For this review, take the finished solid that the model builds, in its own axes (mm). A direction names the side the tool comes from. Coordinates: 2 decimals unless noted, no trailing zeros. Loops run counter-clockwise (first coordinate to the right, second up) from the corner with the lowest first, then second, coordinate; pieces in that order, holes last. Notation, with made-up numbers: (10.25, 49.25) - (31.25, 49.25) arc R7 ccw to (31.25, 61.25) - close; hole circle Ø2 at (45.5, -26). An arc over 180 degrees is marked (long way). Use one line per item in the form item = value. Start each with the question number.
1. Add section B-B on z = 0.3. Give the boundary of the cut face in (x, y).
2. Add section C-C on x = 1.5. Give the boundary of the cut face in (y, z), and give its area (3 significant figures).
3. Add section D-D on y = 1.3. Give the boundary of the cut face in (x, z).
4. To check wall thickness, follow probe 1 along X at (y, z) = (0.9, 3.3); probe 2 along X at (y, z) = (1.05, 3.7); probe 3 along Y at (x, z) = (-0.5, 0.65). State the ranges of each line that lie inside material, in increasing order.
5. For pin 1 Ø1 at (x, z) = (-0.5, 2.5) entering from +Y, flat-tipped, find the tip position at first contact; note if it passes through.
6. Add section A-A on y = 1.9. Give the boundary of the cut face in (x, z).
7. Machinability: for faces 1 (the face through (-1.13, 0.67, 2.46)), 2 (the face through (0, 1, 5)), which of the approach directions +Z, -Z, +X, -X, +Y, -Y give a long, thin tool a straight path to every point of the face, cutting with its end or side? Answer none if there is none.
```python
from build123d import *

# Parameters (mm, degrees)
ESBO_O1_R                  = 0.8
RESSALTO_EXTRUS_O1_DEPTH   = 5
RESSALTO_EXTRUS_O1_2_DEPTH = 5
RESSALTO_EXTRUS_O1_3_DEPTH = 5
RESSALTO_EXTRUS_O1_4_DEPTH = 5
ESBO_O2_R                  = 0.8
ESBO_O2_W                  = 5
ESBO_O2_H                  = 0.5
RESSALTO_EXTRUS_O2_DEPTH   = 1


with BuildPart() as part:
    # Esbo_o1 → Ressalto-extrus_o1 (new body)
    with BuildSketch(Plane.XY):
        with Locations((-3.502077011, 1.3792577)):
            Circle(ESBO_O1_R)
    extrude(amount=RESSALTO_EXTRUS_O1_DEPTH)



with BuildPart() as body_2:
    # Esbo_o1 → Ressalto-extrus_o1 2 (new body)
    with BuildSketch(Plane.XY):
        with Locations((-1.502077011, 1.3792577)):
            Circle(ESBO_O1_R)
    extrude(amount=RESSALTO_EXTRUS_O1_2_DEPTH)


with BuildPart() as body_3:
    # Esbo_o1 → Ressalto-extrus_o1 3 (new body)
    with BuildSketch(Plane.XY):
        with Locations((0.497922989, 1.3792577)):
            Circle(ESBO_O1_R)
    extrude(amount=RESSALTO_EXTRUS_O1_3_DEPTH)


with BuildPart() as body_4:
    # Esbo_o1 → Ressalto-extrus_o1 4 (new body)
    with BuildSketch(Plane.XY):
        with Locations((2.497922989, 1.3792577)):
            Circle(ESBO_O1_R)
    extrude(amount=RESSALTO_EXTRUS_O1_4_DEPTH)


with BuildPart() as part_1:
    add(part.part)

    add(body_2.part)  # Ressalto-extrus_o2 merges body 2

    add(body_3.part)  # Ressalto-extrus_o2 merges body 3

    add(body_4.part)  # Ressalto-extrus_o2 merges body 4
    # Esbo_o2 → Ressalto-extrus_o2 (add)
    with BuildSketch(Plane(origin=(0, 0, 0), x_dir=(-1, 0, 0), z_dir=(0, 0, -1))):
        with Locations((-2.497922989, 1.3792577)):
            Circle(ESBO_O2_R)
        with Locations((3.502077011, 1.3792577)):
            Circle(ESBO_O2_R)
        with Locations((0.502077011, 1.3792577)):
            Rectangle(ESBO_O2_W, ESBO_O2_H)
    extrude(amount=-RESSALTO_EXTRUS_O2_DEPTH)


solid = part_1.part
```
Conclusion:
q1.outline = (-2.74, 1.13) - (-2.26, 1.13) arc R0.8 ccw to (-0.74, 1.13) - (-0.26, 1.13) arc R0.8 ccw to (1.26, 1.13) - (1.74, 1.13) arc R0.8 ccw (long way) to (1.74, 1.63) - (1.26, 1.63) arc R0.8 ccw to (-0.26, 1.63) - (-0.74, 1.63) arc R0.8 ccw to (-2.26, 1.63) - (-2.74, 1.63) arc R0.8 ccw (long way) to start
q2.outline = (1.13, 0) - (1.63, 0) - (1.63, 1) - (1.13, 1) - close
q2.area = 0.500 mm^2
q3.outline = (-4.3, 0) - (3.29, 0) - (3.29, 5) - (1.7, 5) - (1.7, 1) - (1.29, 1) - (1.29, 5) - (-0.3, 5) - (-0.3, 1) - (-0.71, 1) - (-0.71, 5) - (-2.3, 5) - (-2.3, 1) - (-2.71, 1) - (-2.71, 5) - (-4.3, 5) - close
q4.probe_1 = -4.14 to -2.86, -2.14 to -0.86, -0.14 to 1.14, 1.86 to 3.14
q4.probe_2 = -4.23 to -2.77, -2.23 to -0.77, -0.23 to 1.23, 1.77 to 3.23
q4.probe_3 = 1.13 to 1.63
q5.pin_1 = 2.01
q6.outline = (-4.11, 0) - (-2.89, 0) - (-2.89, 5) - (-4.11, 5) - close; (-2.11, 0) - (-0.89, 0) - (-0.89, 5) - (-2.11, 5) - close; (-0.11, 0) - (1.11, 0) - (1.11, 5) - (-0.11, 5) - close; (1.89, 0) - (3.11, 0) - (3.11, 5) - (1.89, 5) - close
q7.face_1 = +Z
q7.face_2 = +Z, +X, -X, +Y, -Y
